Answer from the drawing. Dimensions are ordinates in mm from the lowest x, y and z of the part. A direction names the side the tool comes from. Coordinates: 2 decimals unless noted, no trailing zeros. Order: outer loops, then holes, each group sorted by start corner. A loop starts at its lowest first (then second) coordinate and runs counter-clockwise, first axis right, second up. Notation, with made-up numbers: (24.25, 85.5) -> (72.25, 85.5) arc R17 cw to (72.25, 115.5) -> close; hole circle Ø6 at (18, -12). An arc over 180 degrees is marked (long way). Use CSV: the item, a comma, the result in double quotes.
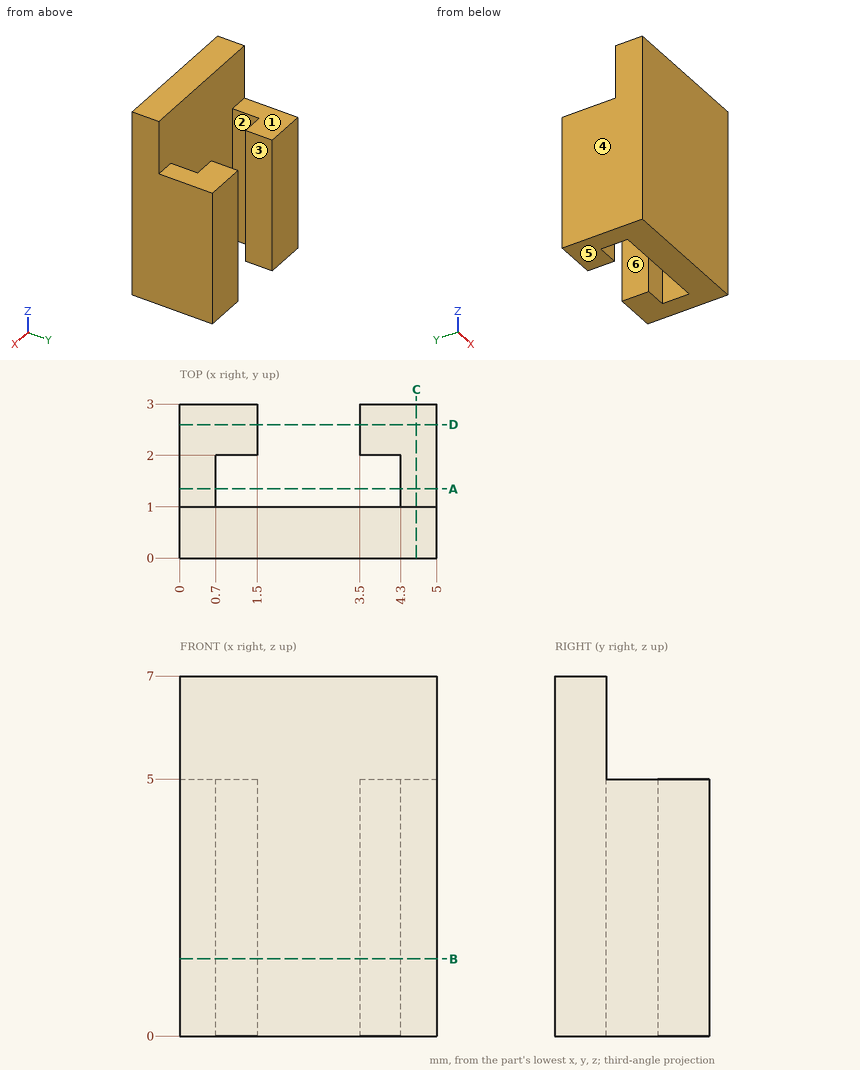
Item 1: A tool of negligible diameter and unlimited length cuts with its end or side. For the marked faces 1, 2 and 3, from which of +Z, -Z, +X, -X, +Y, -Y can it reach the whole face along a straight path? Write none if from no direction.
Return value:
face 1,"+Z, +X, -X, +Y"
face 2,"+Z, -Z"
face 3,"+Z, -Z, +Y"
Item 2: Straight lines are drawn through the part: line 1 along X through (y, z) = (2.4, 4.5); line 2 along Y through (x, z) = (3.9, 2.5); line 3 along X through (y, z) = (1.8, 1). For each, find the intervals that lie inside material, in ascending order.
Return value:
line 1,"x = 0 to 1.5, 3.5 to 5"
line 2,"y = 0 to 1, 2 to 3"
line 3,"x = 0 to 0.7, 4.3 to 5"
Item 3: Find section B-B, the plane z = 1.5. Give the vertices of the cut face in (x, y).
Return value:
outline,"(0, 0) -> (5, 0) -> (5, 3) -> (3.5, 3) -> (3.5, 2) -> (4.3, 2) -> (4.3, 1) -> (0.7, 1) -> (0.7, 2) -> (1.5, 2) -> (1.5, 3) -> (0, 3) -> close"
Item 4: Find section C-C, the plane x = 4.6. Give the vertices of the cut face in (y, z).
Return value:
outline,"(0, 0) -> (3, 0) -> (3, 5) -> (1, 5) -> (1, 7) -> (0, 7) -> close"
Item 5: Each of these flat-tipped pins is pushed along its axis until it touches: P1, Ø1.5, axis at x = 2, z = 6.5, coming from the +Y side; P2, Ø1.2, axis at x = 0.5, y = 2, coming from the +Z side. Where does it stop, or does it pass through?
Return value:
P1,"stops at y = 1"
P2,"stops at z = 5"
Item 6: Find section D-D, the plane y = 2.6. Give the vertices of the cut face in (x, z).
Return value:
outline,"(0, 0) -> (1.5, 0) -> (1.5, 5) -> (0, 5) -> close; (3.5, 0) -> (5, 0) -> (5, 5) -> (3.5, 5) -> close"
Item 7: Find section A-A, the plane y = 1.35. Give the vertices of the cut face in (x, z), then the cut area to 3 significant figures.
Return value:
outline,"(0, 0) -> (0.7, 0) -> (0.7, 5) -> (0, 5) -> close; (4.3, 0) -> (5, 0) -> (5, 5) -> (4.3, 5) -> close"
area,"7.00 mm^2"
Item 8: The mould has two halves that part along X. Classify the marked faces 4, 5 and 6: +X half, -X half, draft (parallel to the pull), parting line (faces both ways), or undercut.
Return value:
face 4,"-X half"
face 5,"draft"
face 6,"undercut"
